Check sheet for the modelled part. Datum: model origin and axes. Units: mm. A direction names the side the tool comes from. Give positions to 0.01 mm unless a question says otherwise; leave off trailing zeros. Loops run counter-clockwise (first coordinate to the right, second up) from the corner with the lowest first, then second, coordinate; pieces in that order, holes last. Notation, with made-up numbers: M -9,-28 L 39,-28 A26 ccw 39,8 Z; hole C 14.5,29.25 d6. An arc over 180 degrees is marked long. Use one line per item in the form item = value.
from build123d import *

# Parameters (mm, degrees)
SKETCH1_W               = 40
SKETCH1_H               = 160
BOSS_EXTRUDE1_DEPTH     = 3.175
M4_5_THROUGH_DEPTH      = 6.35
M4_5_THROUGH_DEPTH_BACK = 3.175
SKETCH3_R               = 2.75
SKETCH3_R_2             = 2.25
SKETCH4_R               = 1.5
M3_DRILL_DEPTH          = 8
SKETCH5_R               = 2.25
M4_THROUGH_DEPTH        = 6.35
SKETCH6_W               = 40
SKETCH6_H               = 30.2375
CUT_EXTRUDE1_DEPTH      = 6.35


with BuildPart() as part:
    # Sketch1 → Boss-Extrude1 (new, symmetric)
    with BuildSketch(Plane(origin=(0, 0, 0), x_dir=(1, 0, 0), z_dir=(0, 1, 0))):
        Rectangle(SKETCH1_W, SKETCH1_H)
    extrude(amount=BOSS_EXTRUDE1_DEPTH, both=True)

    # Sketch3 → M4/5_through (cut, two sides: drawn at the far end of the back side and taken through both)
    with BuildSketch(Plane(origin=(0, 0, 0), x_dir=(1, 0, 0), z_dir=(0, 1, 0)).offset(-M4_5_THROUGH_DEPTH_BACK)):
        with Locations(Location((12, 75.2375, 0), (0, 0, 270))):
            Circle(SKETCH3_R)
        with Locations(Location((12, 50.2375, 0), (0, 0, 270))):
            Circle(SKETCH3_R_2)
        with Locations(Location((-12, 50.2375, 0), (0, 0, 270))):
            Circle(SKETCH3_R_2)
        with Locations(Location((-12, 75.2375, 0), (0, 0, 270))):
            Circle(SKETCH3_R)
        with Locations(Location((-12, -44.7625, 0), (0, 0, 270))):
            Circle(SKETCH3_R_2)
        with Locations(Location((12, -44.7625, 0), (0, 0, 270))):
            Circle(SKETCH3_R_2)
    extrude(amount=M4_5_THROUGH_DEPTH + M4_5_THROUGH_DEPTH_BACK, mode=Mode.SUBTRACT)

    # Sketch4 → M3_DRILL (cut)
    with BuildSketch(Plane(origin=(0, 0, -80), x_dir=(-1, 0, 0), z_dir=(0, 0, -1))):
        Circle(SKETCH4_R)
    extrude(amount=-M3_DRILL_DEPTH, mode=Mode.SUBTRACT)

    # Sketch5 → M4_through (cut)
    with BuildSketch(Plane(origin=(0, 3.175, 0), x_dir=(1, 0, 0), z_dir=(0, 1, 0))):
        with Locations(Location((-15.2375, -27.6625, 0), (0, 0, 270))):
            Circle(SKETCH5_R)
        with Locations(Location((15.2375, -27.6625, 0), (0, 0, 270))):
            Circle(SKETCH5_R)
        with Locations(Location((15.2375, 33.1375, 0), (0, 0, 270))):
            Circle(SKETCH5_R)
        with Locations(Location((-15.2375, 33.1375, 0), (0, 0, 270))):
            Circle(SKETCH5_R)
    extrude(amount=-M4_THROUGH_DEPTH, mode=Mode.SUBTRACT)

    # Sketch6 → Cut-Extrude1 (cut)
    with BuildSketch(Plane(origin=(0, 3.175, 0), x_dir=(1, 0, 0), z_dir=(0, 1, 0))):
        with Locations((0, -64.88125)):
            Rectangle(SKETCH6_W, SKETCH6_H)
    extrude(amount=-CUT_EXTRUDE1_DEPTH, mode=Mode.SUBTRACT)


solid = part.part
1) Set-up check for faces 5 (the face through (12.121, -0.044, -77.985)), 6 (the face through (0, 0, -72)): record each of +Z, -Z, +X, -X, +Y, -Y from which the full face is reachable in a straight line by a thin tool's end or side.
Evaluation:
face_5 = +Y, -Y
face_6 = -Z
2) Scan lines: line 1 (Z direction, x = -15, y = 0); line 2 (Z direction, x = 12, y = 0); line 3 (X direction, y = -1, z = 44.5). Record each from-to range of solid material in increasing order.
Evaluation:
line_1 = -80 to -35.37, -30.9 to 25.43, 29.9 to 49.76
line_2 = -80 to -77.99, -72.49 to -52.49, -47.99 to 42.51, 47.01 to 49.76
line_3 = -20 to -14.23, -9.77 to 9.77, 14.23 to 20
3) Release check for a two-part mould opening along X. For faces 1 (the face through (-20, 0, -14)), 2 (the face through (0, -3.175, -16)), 3 (the face through (15.336, 0.044, -35.385)), 4 (the face through (20, 0, -14)) record: pulls with the +X half, pulls with the -X half, needs draft (parallel to the pull), parting line crosses it, or undercut.
Evaluation:
face_1 = pulls with the -X half
face_2 = needs draft
face_3 = undercut
face_4 = pulls with the +X half
4) Section check B-B (y = 0). State how many separate pieces and enclosed holes the cut face has, then the cut area to 3 significant figures.
Evaluation:
separate_pieces = 1
enclosed_holes = 10
area = 4,990 mm^2
5) Depth check by flat-ended pin: pin 1 Ø0.9 at (x, y) = (0, 0.5) entering from -Z. Enter the tip coordinate at first touch or a pass-through.
Evaluation:
pin_1 = -72
6) Section check A-A (x = 0). Record the cut outline in (y, z) (1 decimal).
Evaluation:
outline = M -3.2,-80 L -1.5,-80 L -1.5,-72 L 1.5,-72 L 1.5,-80 L 3.2,-80 L 3.2,49.8 L -3.2,49.8 Z
